The model under review builds one solid part; all positions refer to its coordinate system, in mm. Face numbers are marked on the shaded views. A direction names the side the tool comes from. Round coordinates to 2 decimals unless told otherwise and drop trailing zeros. Write each loop counter-clockwise with the first axis right and the second up, starting at its lowest first coordinate (ties: lowest second). Pieces come first, ordered by that corner, then holes. Notation, with made-up numbers: M 29.25,76 L 88.25,76 A30 ccw 88.25,108 Z; hole C -31.75,24 d2. An arc over 180 degrees is marked long. Write item = value, one per line. Start each with the question number.
Item 1: For pin 1 Ø1 at (x, y) = (18.5, 13.5) entering from -Z, flat-tipped, find the tip position at first contact; note if it passes through.
Item 2: Take a section at D-D, the plane z = 11. Give the boundary of the cut face in (x, y).
Item 3: Take a section at A-A, the plane x = 6. Give the boundary of the cut face in (y, z), plus the area to 3 significant figures.
Item 4: The part is to be moulded in two halves that separate along Y. For the marked faces 1, 2 and 3, say which applies: +Y half, -Y half, draft (parallel to the pull), parting line (faces both ways), or undercut.
Item 5: To check wall thickness, follow line 1 along Y through (x, z) = (4.5, 15); line 2 along Z through (x, y) = (4.75, 16.5); line 3 along Y through (x, z) = (20, 3). State the ranges of each line that lie inside material, in increasing order.
Item 6: Take a section at C-C, the plane x = 16.25. Give the boundary of the cut face in (y, z).
Item 7: Tool access review of the marked faces 4 and 5: name each direction out of +Z, -Z, +X, -X, +Y, -Y from which nothing blocks a thin tool from reaching the whole face with its end or side.
Item 8: Take a section at B-B, the plane z = 15. Give the boundary of the cut face in (x, y), plus the area to 3 significant figures.
Autodesk Fusion 360 part; units mm, degrees
sketch "Esboço1" plane through (0, 0, 0) normal (0, 0, 1) x (1, 0, 0)
  line L0 (1.9999, 62) -> (21, 62)
  line L1 (21, 62) -> (21, 54)
  line L2 (21, 54) -> (13, 54)
  line L3 (13, 54) -> (13, 38)
  line L4 (13, 38) -> (21, 38)
  arc A0 (21, 33) -> (21, 11) centre (21, 22) ccw
  line L5 (21, 11) -> (21, 3)
  line L6 (2, 3) -> (2, 62)
  line L7 (2, 3) -> (21, 3)
  line L8 (21, 33) -> (21, 38)
  line L9 (1.9999, 62) -> (2, 62)
  dimension "d1" = 11
  dimension "d2" = 16
  dimension "d3" = 8
  dimension "d5" = 8
  dimension "d8" = 8
  dimension "d10" = 8
  dimension "d35" = 5
  dimension "d36" = 19
extrude "Extrusão1" add sketch "Esboço1" along normal blind 30
hole "Furo2" at (2, 16.5, 15) direction (1, 0, 0) diameter 4 depth 21 tip angle 180
hole "Furo3" at (2, 48, 15) direction (1, 0, 0) diameter 4 depth 21 tip angle 180
fillet "Arredondamento4" radius 1.5 8 edges at (11.5, 62, 30) (2, 62, 15) (2, 32.5, 30) (2, 32.5, 0) (2, 3, 15) (11.5, 3, 0) (11.5, 3, 30) (11.5, 62, 0)
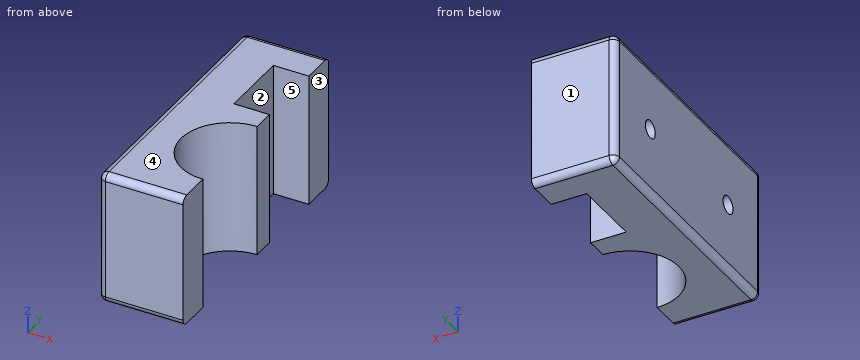
Response values:
q1.pin_1 = through
q2.outline = M 2,4.5 A1.5 ccw 3.5,3 L 21,3 L 21,11 A11 cw 21,33 L 21,38 L 13,38 L 13,54 L 21,54 L 21,62 L 3.5,62 A1.5 ccw 2,60.5 Z
q3.outline = M 3,1.5 A1.5 ccw 4.5,0 L 60.5,0 A1.5 ccw 62,1.5 L 62,28.5 A1.5 ccw 60.5,30 L 4.5,30 A1.5 ccw 3,28.5 Z; hole C 16.5,15 d4; hole C 48,15 d4
q3.area = 1,740 mm2
q4.face_1 = +Y half
q4.face_2 = undercut
q4.face_3 = draft
q5.line_1 = 3 to 14.5, 18.5 to 46, 50 to 62
q5.line_2 = 0 to 13, 17 to 30
q5.line_3 = 3 to 11.05, 32.95 to 38, 54 to 62
q6.outline = M 3,1.5 A1.5 ccw 4.5,0 L 12.08,0 L 12.08,30 L 4.5,30 A1.5 ccw 3,28.5 Z; M 31.92,0 L 38,0 L 38,30 L 31.92,30 Z; M 54,0 L 60.5,0 A1.5 ccw 62,1.5 L 62,28.5 A1.5 ccw 60.5,30 L 54,30 Z
q7.face_4 = +Z, +X, -X, +Y, -Y
q7.face_5 = +Z, -Z, +X
q8.outline = M 2,4.5 A1.5 ccw 3.5,3 L 21,3 L 21,11 A11 cw 12.95,14.5 L 2,14.5 Z; M 2,18.5 L 10.57,18.5 A11 cw 21,33 L 21,38 L 13,38 L 13,46 L 2,46 Z; M 2,50 L 13,50 L 13,54 L 21,54 L 21,62 L 3.5,62 A1.5 ccw 2,60.5 Z
q8.area = 720 mm2
